The listing builds one solid part. Answer for the finished solid, in the listing's coordinates (mm). A direction names the side the tool comes from. Round coordinates to 2 decimals unless told otherwise and drop trailing zeros. Order: outer loops, then holes, each group sorted by start corner. A loop starts at its lowest first (then second) coordinate and runs counter-clockwise, first axis right, second up. Notation, with made-up numbers: M 57.25,79.25 L 114.25,79.25 A18 cw 114.25,112.25 Z; hole C 4.25,63.25 d7. An arc over 180 degrees is marked long. Put each result on its own line as item: value. Start each with the question number.
1. Which of the six approach directions +Z, -Z, +X, -X, +Y, -Y give full straight-line access (tool end or side, diameter ignored) to faces 4 (the face through (-9, 1.6, 8)), 5 (the face through (0, 8, 8))?
2. The mould has two halves that part along Z. Classify faces 1 (the face through (-1.6, 9, 8)), 2 (the face through (-1, 4, 15.5)), 3 (the face through (-14.234, 0.811, 9.271)): +Z half, -Z half, draft (parallel to the pull), parting line (faces both ways), or undercut.
3. Consider line 1 (Y direction, x = -0.75, z = 7.75); line 2 (X direction, y = 0.5, z = 7.75); line 3 (Z direction, x = -12.25, y = 1.15). Determine where each line is inside the solid, lowest interval first.
4. The part is cut by section D-D (z = 11.5). Give the vertices of the cut face in (x, y), then the cut area to 3 significant figures.
5. The part is cut by section C-C (z = 7.25). Give the vertices of the cut face in (x, y), then the cut area to 3 significant figures.
6. Each of these flat-tipped pins is pushed along its axis until it touches: pin 1 Ø6 at (x, z) = (-2.5, 6) entering from -Y; pin 2 Ø8 at (x, z) = (-9.5, 8.5) entering from +Y; pin 3 Ø4 at (y, z) = (2.5, 5.5) entering from -X; pin 4 Ø6 at (y, z) = (16.5, 7.5) entering from -X. Where does it stop, or does it pass through?
7. The part is cut by section A-A (y = 11). Give the vertices of the cut face in (x, z), then the cut area to 3 significant figures.
8. The part is cut by section B-B (x = -11). Give the vertices of the cut face in (y, z), then the cut area to 3 significant figures.
from build123d import *

# Parameters (mm, degrees)
EXTRUDE_1_DEPTH     = 15.5
CUT_EXTRUDE_1_DEPTH = 15.5
CUT_EXTRUDE_2_DEPTH = 15.5
SKETCH_4_R          = 2.5
CUT_EXTRUDE_3_DEPTH = 15.5
SKETCH_5_R          = 2.5
CUT_EXTRUDE_4_DEPTH = 15.5


with BuildPart() as part:
    # 草图1 → 凸台-拉伸1 (new body)
    with BuildSketch(Plane.XY):
        Polygon((0, 0), (-20, 0), (-20, 1.6), (-1.6, 1.6), (-1.6, 20), (0, 20), align=None)
    extrude(amount=EXTRUDE_1_DEPTH)

    # 草图2 → 切除-拉伸1 (cut)
    with BuildSketch(Plane.ZY.offset(1.6)):
        with BuildLine():
            Line((0, 20), (0, 12.25))
            ThreePointArc((0, 12.25), (2.269922446, 17.730077554), (7.75, 20))
            Line((7.75, 20), (0, 20))
        make_face()
        with BuildLine():
            ThreePointArc((7.75, 20), (13.230077554, 17.730077554), (15.5, 12.25))
            Line((15.5, 12.25), (15.5, 20))
            Line((15.5, 20), (7.75, 20))
        make_face()
    extrude(amount=-CUT_EXTRUDE_1_DEPTH, mode=Mode.SUBTRACT)

    # 草图3 → 切除-拉伸2 (cut)
    with BuildSketch(Plane(origin=(0, 1.6, 0), x_dir=(1, 0, 0), z_dir=(0, 1, 0))):
        with BuildLine():
            ThreePointArc((-12.25, -15.5), (-17.730077554, -13.230077554), (-20, -7.75))
            Line((-20, -7.75), (-20, -15.5))
            Line((-20, -15.5), (-12.25, -15.5))
        make_face()
        with BuildLine():
            ThreePointArc((-20, -7.75), (-17.730077554, -2.269922446), (-12.25, 0))
            Line((-12.25, 0), (-20, 0))
            Line((-20, 0), (-20, -7.75))
        make_face()
    extrude(amount=-CUT_EXTRUDE_2_DEPTH, mode=Mode.SUBTRACT)

    # 草图4 → 切除-拉伸3 (cut)
    with BuildSketch(Plane.ZY.offset(1.6)):
        with Locations((7.75, 12.25)):
            Circle(SKETCH_4_R)
    extrude(amount=-CUT_EXTRUDE_3_DEPTH, mode=Mode.SUBTRACT)

    # 草图5 → 切除-拉伸4 (cut)
    with BuildSketch(Plane(origin=(0, 1.6, 0), x_dir=(1, 0, 0), z_dir=(0, 1, 0))):
        with Locations((-12.25, -7.75)):
            Circle(SKETCH_5_R)
    extrude(amount=-CUT_EXTRUDE_4_DEPTH, mode=Mode.SUBTRACT)


solid = part.part
Resolved:
1. face 4: +Z, -Z, -X, +Y
1. face 5: +Z, -Z, +X, +Y, -Y
2. face 1: draft
2. face 2: +Z half
2. face 3: undercut
3. line 1: 0 to 9.75, 14.75 to 20
3. line 2: -20 to -14.75, -9.75 to 0
3. line 3: 0 to 5.25, 10.25 to 15.5
4. outline: M -19.03,0 L 0,0 L 0,19.03 L -1.6,19.03 L -1.6,1.6 L -19.03,1.6 Z
4. area: 58.3 mm2
5. outline: M -19.98,0 L -14.7,0 L -14.7,1.6 L -19.98,1.6 Z; M -9.8,0 L 0,0 L 0,9.8 L -1.6,9.8 L -1.6,1.6 L -9.8,1.6 Z; M -1.6,14.7 L 0,14.7 L 0,19.98 L -1.6,19.98 Z
5. area: 45.7 mm2
6. pin 1: y = 0
6. pin 2: y = 1.6
6. pin 3: x = -19.99
6. pin 4: x = -1.6
7. outline: M -1.6,0 L 0,0 L 0,5.58 L -1.6,5.58 Z; M -1.6,9.92 L 0,9.92 L 0,15.5 L -1.6,15.5 Z
7. area: 17.9 mm2
8. outline: M 0,0 L 1.6,0 L 1.6,5.58 L 0,5.58 Z; M 0,9.92 L 1.6,9.92 L 1.6,15.5 L 0,15.5 Z
8. area: 17.9 mm2
